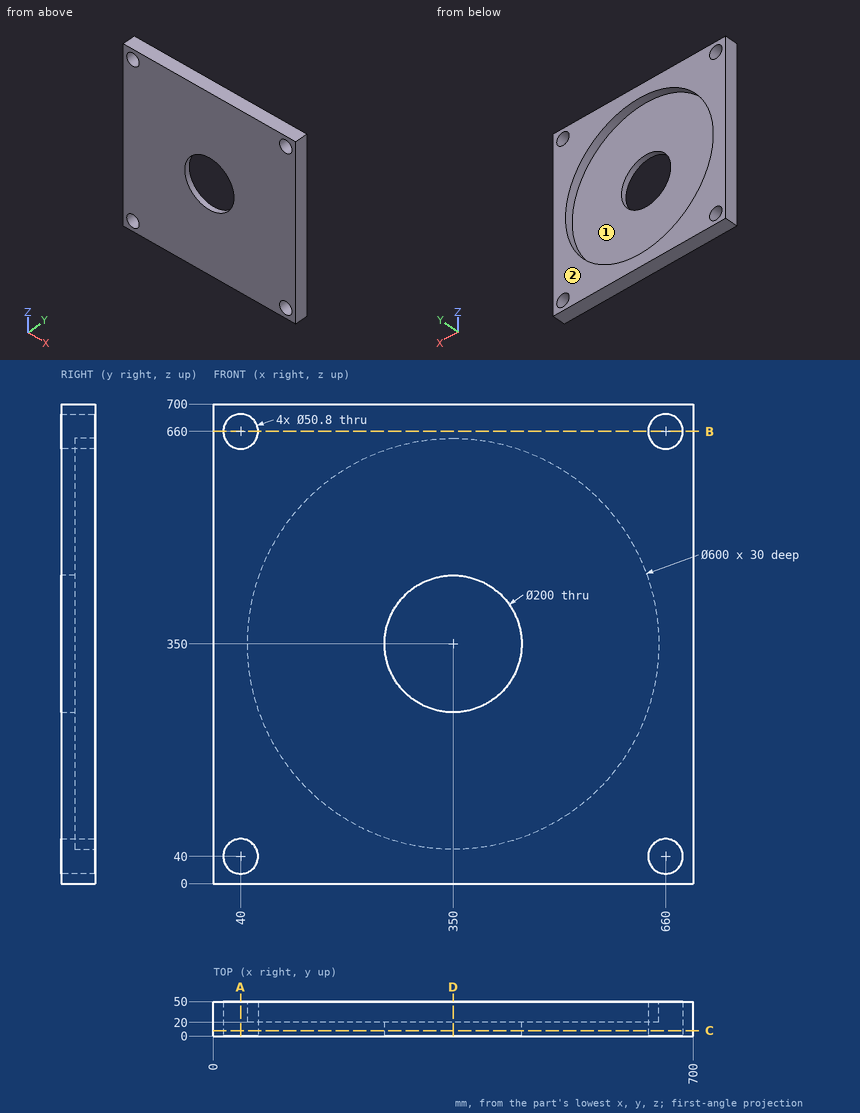
Input: dimensioned drawing with shaded views. Units: mm. Origin: part minimum x, y, z. Give positions to 0.01 mm unless a question says otherwise; leave off trailing zeros. Write each loop counter-clockwise with the first axis right and the second up, starting at its lowest first coordinate (ties: lowest second). Pieces come first, ordered by that corner, then holes.
1. Section query A-A (x = 40). Return the cut outline in (y, z).
2. Section query D-D (x = 350). Return the cut outline in (y, z).
3. First-contact query: pin 1 (8 mm diameter, centred on y = 24.5, z = 498.5, fed in from -X); pin 2 (1.5 mm diameter, centred on x = 191, z = 271.5, fed in from +Y). Flat tips, straight axial feed; report the tip coordinate or a pass-through.
4. Section query C-C (y = 8). Return the cut outline in (x, z), then the cut area to 3 significant figures.
5. Pull-direction query (Z, two-part tool) for the marked faces 1 and 2; classes: +Z half, -Z half, draft (parallel to the pull), parting line (faces both ways), or undercut.
6. Section query B-B (z = 660). Return the cut outline in (x, y), then the cut area to 3 significant figures.
7. Material intervals for line 1 along Z through (x, y) = (660, 38); line 2 along X through (y, z) = (9, 350), sorted ascending.
Output values:
1. outline: (0, 0) - (50, 0) - (50, 14.6) - (0, 14.6) - close; (0, 65.4) - (50, 65.4) - (50, 634.6) - (0, 634.6) - close; (0, 685.4) - (50, 685.4) - (50, 700) - (0, 700) - close
2. outline: (0, 0) - (50, 0) - (50, 50) - (20, 50) - (20, 250) - (0, 250) - close; (0, 450) - (20, 450) - (20, 650) - (50, 650) - (50, 700) - (0, 700) - close
3. pin 1: stops at x = 0
3. pin 2: stops at y = 20
4. outline: (0, 0) - (700, 0) - (700, 700) - (0, 700) - close; hole circle Ø50.8 at (40, 40); hole circle Ø50.8 at (40, 660); hole circle Ø200 at (350, 350); hole circle Ø50.8 at (660, 40); hole circle Ø50.8 at (660, 660)
4. area: 450,000 mm2
5. face 1: undercut
5. face 2: draft
6. outline: (0, 0) - (14.6, 0) - (14.6, 50) - (0, 50) - close; (65.4, 0) - (634.6, 0) - (634.6, 50) - (65.4, 50) - close; (685.4, 0) - (700, 0) - (700, 50) - (685.4, 50) - close
6. area: 29,900 mm2
7. line 1: z = 0 to 14.6, 65.4 to 634.6, 685.4 to 700
7. line 2: x = 0 to 250, 450 to 700
